The figure shows three views and two pictorial views of one solid part (mm, origin at its lowest corner). Answer the questions. A direction names the side the tool comes from. Coordinates: 2 decimals unless noted, no trailing zeros. Loops run counter-clockwise (first coordinate to the right, second up) from the corner with the lowest first, then second, coordinate; pieces in that order, holes last. Notation, with made-up numbers: M -1,36.5 L 22,36.5 A33 cw 22,72.5 Z; hole C -29.5,73.25 d10. An arc over 180 degrees is marked long. Return JSON: item names as keys, results as strings. Group by question number.
1. Straight lines are drawn through the part: L1, parallel to Z at x = 40, y = 2.7; L2, parallel to X at y = 10, z = 4.25; L3, parallel to X at y = 10.75, z = 3. For each, find the intervals that lie inside material, in ascending order. Write a range as from..to.
2. Section A-A (y = 10) is taken. Write down the section's boundary in (x, z).
3. Section D-D (y = 13.75) is taken. Write down the section's boundary in (x, z), then the cut area to 3 significant figures.
4. Section B-B (x = 40) is taken. Write down the section's boundary in (y, z).
5. Which of the six approach directions +Z, -Z, +X, -X, +Y, -Y give full straight-line access (tool end or side, diameter ignored) to the marked faces 4, 5 and 6?
6. The mould has two halves that part along X. Classify the marked faces 1, 2 and 3: pulls with the +X half, pulls with the -X half, needs draft (parallel to the pull), parting line crosses it, or undercut.
7. Given P1, Ø10, axis at x = 69.5, y = 8.5, coming from the +Z side; P2, Ø12, axis at y = 16, z = 35.5, coming from the +X side; P3, Ø10, axis at y = 8, z = 27, coming from the -X side, each flat-ended and moving along its own axis, determine where each tip first touches the part or whether it passes through.
8. Section C-C (z = 25) is taken. Write down the section's boundary in (x, y), then the cut area to 3 significant figures.
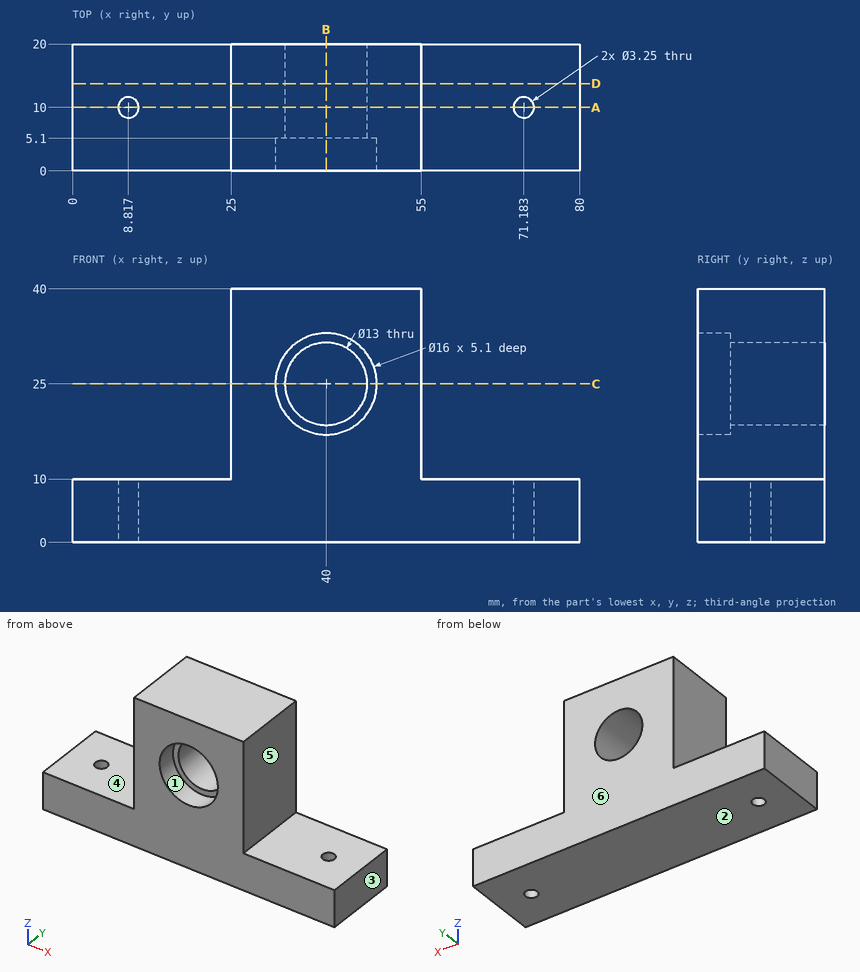
Worked out:
{
 "1": {"L1": "0..17, 33..40", "L2": "0..7.19, 10.44..69.56, 72.81..80", "L3": "0..7.38, 10.26..69.74, 72.62..80"},
 "2": {"outline": "M 0,0 L 7.19,0 L 7.19,10 L 0,10 Z; M 10.44,0 L 69.56,0 L 69.56,10 L 55,10 L 55,40 L 25,40 L 25,10 L 10.44,10 Z; M 72.81,0 L 80,0 L 80,10 L 72.81,10 Z; hole C 40,25 d13"},
 "3": {"outline": "M 0,0 L 80,0 L 80,10 L 55,10 L 55,40 L 25,40 L 25,10 L 0,10 Z; hole C 40,25 d13", "area": "1,570 mm^2"},
 "4": {"outline": "M 0,0 L 20,0 L 20,18.5 L 5.1,18.5 L 5.1,17 L 0,17 Z; M 0,33 L 5.1,33 L 5.1,31.5 L 20,31.5 L 20,40 L 0,40 Z"},
 "5": {"face 4": "+Z, -X, +Y, -Y", "face 5": "+Z, +X, +Y, -Y", "face 6": "+Z, -Z, +X, -X, +Y"},
 "6": {"face 1": "undercut", "face 2": "needs draft", "face 3": "pulls with the +X half"},
 "7": {"P1": "z = 10", "P2": "x = 55", "P3": "x = 25"},
 "8": {"outline": "M 25,0 L 32,0 L 32,5.1 L 33.5,5.1 L 33.5,20 L 25,20 Z; M 46.5,5.1 L 48,5.1 L 48,0 L 55,0 L 55,20 L 46.5,20 Z", "area": "325 mm^2"}
}
